```python
from build123d import *

# Parameters (mm, degrees)
SKETCH_W     = 12
SKETCH_H     = 12
PAD_DEPTH    = 3.4
SKETCH001_R  = 4.75
PAD001_DEPTH = 11.1
SKETCH002_R  = 3.571924
POCKET_DEPTH = 1
SKETCH003_R  = 0.55
PAD002_DEPTH = 4.572


with BuildPart() as part:
    # Sketch → Pad (new body)
    with BuildSketch(Plane.XY):
        Rectangle(SKETCH_W, SKETCH_H)
    extrude(amount=PAD_DEPTH)

    # Sketch001 (on Face6 of Pad) → Pad001 (join)
    with BuildSketch(Plane.XY.offset(3.4)):
        Circle(SKETCH001_R)
    extrude(amount=PAD001_DEPTH)

    # Sketch002 (on Face4 of Pad001) → Pocket (cut)
    with BuildSketch(Plane(origin=(0, 0, 0), x_dir=(1, 0, 0), z_dir=(0, 0, -1))):
        Circle(SKETCH002_R)
    extrude(amount=-POCKET_DEPTH, mode=Mode.SUBTRACT)

    # Sketch003 (on Face9 of Pocket) → Pad002 (join)
    with BuildSketch(Plane(origin=(0, 0, 1), x_dir=(1, 0, 0), z_dir=(0, 0, -1))):
        Circle(SKETCH003_R)
        with Locations((-5, 5)):
            Circle(SKETCH003_R)
        with Locations((5, 5)):
            Circle(SKETCH003_R)
        with Locations((5, -5)):
            Circle(SKETCH003_R)
        with Locations((-5, -5)):
            Circle(SKETCH003_R)
    extrude(amount=PAD002_DEPTH)


solid = part.part
```
Could you check a few things on this model? Use its own coordinates, in mm. A direction names the side the tool comes from. Give positions to 0.01 mm unless a question says otherwise; leave off trailing zeros. Write each loop counter-clockwise with the first axis right and the second up, starting at its lowest first coordinate (ties: lowest second). Pieces come first, ordered by that corner, then holes. Notation, with made-up numbers: (-35, 16.5) -> (-15, 16.5) arc R37 cw to (-15, 54.5) -> close; hole circle Ø2 at (11.5, 47.25). An arc over 180 degrees is marked (long way). Write each question's results on one line, items separated by ' | '.
1. I want a section at B-B, the plane x = 0. Write out the boundary of the cut face in (y, z).
Check sheet entries:
outline: (-6, 0) -> (-3.57, 0) -> (-3.57, 1) -> (-0.55, 1) -> (-0.55, -3.57) -> (0.55, -3.57) -> (0.55, 1) -> (3.57, 1) -> (3.57, 0) -> (6, 0) -> (6, 3.4) -> (4.75, 3.4) -> (4.75, 14.5) -> (-4.75, 14.5) -> (-4.75, 3.4) -> (-6, 3.4) -> close
2. I want a section at A-A, the plane y = -5. Write out the boundary of the cut face in (x, z).
Check sheet entries:
outline: (-6, 0) -> (-5.55, 0) -> (-5.55, -3.57) -> (-4.45, -3.57) -> (-4.45, 0) -> (4.45, 0) -> (4.45, -3.57) -> (5.55, -3.57) -> (5.55, 0) -> (6, 0) -> (6, 3.4) -> (-6, 3.4) -> close
3. Will these pins go through, and if not, where does the flat tip stop? pin 1 Ø2 at (y, z) = (-3.5, 5) entering from -X; pin 2 Ø6 at (x, z) = (-1, 9) entering from -Y; pin 3 Ø1 at (x, y) = (4, -1) entering from -Z.
Check sheet entries:
pin 1: stops at x = -4.04 | pin 2: stops at y = -4.75 | pin 3: stops at z = 0
4. On a 3-axis mill with a long thin cutter (end or side, diameter ignored), from which of +Z, -Z, +X, -X, +Y, -Y can I reach the whole of each face in a straight line? I mean faces 4 (the flat face through (0, -6, 2)), 5 (the cylindrical face through (2.192, -4.214, 8.872)), 6 (the cylindrical face through (-4.49, 5.21, -1.76)). Say none if no direction works.
Check sheet entries:
face 4: +Z, -Z, +X, -X, -Y | face 5: +Z | face 6: -Z
5. If we mould it in two halves opening along X, with no side actions, what happens to faces 1 (the flat face through (-5, 5, -3.572)), 2 (the flat face through (-6, 0, 2)), 3 (the cylindrical face through (3.3, 1.37, 0.49))? For each: released by +X, released by -X, zero draft, split by the parting line, or undercut.
Check sheet entries:
face 1: zero draft | face 2: released by -X | face 3: undercut
6. I need wall thicknesses on L1, parallel to Y at x = 0, z = 0.7; L2, parallel to Z at x = -3.5, y = 1. Which ranges of each line are inside material? Lowest first, please.
Check sheet entries:
L1: y = -6 to -3.57, -0.55 to 0.55, 3.57 to 6 | L2: z = 0 to 14.5
7. I want a section at C-C, the plane z = 5. Write out the boundary of the cut face in (x, y).
Check sheet entries:
outline: circle Ø9.5 at (0, 0)
